from build123d import *

# Parameters (mm, degrees)
F0_W      = 57.15
F0_H      = 31.75
F1_DEPTH  = 38.1
F2_DEPTH  = 12.7
F4_DEPTH  = 12.7
F6_DEPTH  = 12.7
F8_DEPTH  = 38.101
F9_DEPTH  = 6.35
F10_DEPTH = 6.35
F11_DEPTH = 6.35
F12_DEPTH = 6.35


with BuildPart() as f1:
    # F0 (on Front) → F1 (new body)
    with BuildSketch(Plane.XZ):
        with Locations((28.575, 15.875)):
            Rectangle(F0_W, F0_H)
    extrude(amount=F1_DEPTH)

    # F2 (add): a face of the model
    f2_faces = [f1.faces().sort_by_distance(p)[0] for p in [
        (28.575, -38.1, 15.875),
    ]]
    extrude(f2_faces, amount=F2_DEPTH)

    # F3 (on face) → F4 (cut)
    with BuildSketch(Plane.XZ.offset(50.8)):
        Polygon((57.15, 31.75), (23.6781723797, 31.75), (35.8164422214, 0), (57.15, 0), align=None)
    extrude(amount=-F4_DEPTH, mode=Mode.SUBTRACT)

    # F5 (on face) → F6 (cut)
    with BuildSketch(Plane(origin=(0, 0, 0), x_dir=(-1, 0, 0), z_dir=(0, 1, 0))):
        Polygon((-33.819206059, 0), (-23.4500579536, 31.75), (-57.15, 31.75), (-57.15, 0), align=None)
    extrude(amount=-F6_DEPTH, mode=Mode.SUBTRACT)

    # F7 (on face) → F8 (cut, through all)
    with BuildSketch(Plane.XZ.offset(38.1)):
        Polygon((57.15, 31.75), (43.5097105801, 31.75), (57.15, 0), align=None)
    extrude(amount=-F8_DEPTH, mode=Mode.SUBTRACT)

    # F9 (cut): a face of the model
    f9_faces = [f1.faces().sort_by_distance(p)[0] for p in [
        (40.1169646518, -38.1, 15.6819192663),
    ]]
    extrude(f9_faces, amount=-F9_DEPTH, mode=Mode.SUBTRACT)

    # F10 (cut): a face of the model
    f10_faces = [f1.faces().sort_by_distance(p)[0] for p in [
        (39.6330799675, -12.7, 15.4760691102),
    ]]
    extrude(f10_faces, amount=-F10_DEPTH, mode=Mode.SUBTRACT)

    # F11 (cut): a face of the model
    f11_faces = [f1.faces().sort_by_distance(p)[0] for p in [
        (14.4737687914, 0, 14.9168931282),
    ]]
    extrude(f11_faces, amount=-F11_DEPTH, mode=Mode.SUBTRACT)

    # F12 (cut): a face of the model
    f12_faces = [f1.faces().sort_by_distance(p)[0] for p in [
        (15.0800275041, -50.8, 14.7953782839),
    ]]
    extrude(f12_faces, amount=-F12_DEPTH, mode=Mode.SUBTRACT)


solid = f1.part
Input: part model. Units: mm. Frame: model coordinates. A direction names the side the tool comes from. Coordinates: 2 decimals unless noted, no trailing zeros. Loops run counter-clockwise (first coordinate to the right, second up) from the corner with the lowest first, then second, coordinate; pieces in that order, holes last.
(1) Section D-D on y = -33. Return the cut outline in (x, z), then the cut area to 3 significant figures.
(2) Section A-A on z = 12.5. Return the cut outline in (x, y), then the cut area to 3 significant figures.
(3) Section C-C on z = 24.5. Return the cut outline in (x, y), then the cut area to 3 significant figures.
(4) First-contact query: pin 1 Ø5 at (x, y) = (48.5, -35.5) entering from -Z; pin 2 Ø9.5 at (x, z) = (41.5, 17.5) entering from +Y; pin 3 Ø2 at (y, z) = (-26, 26) entering from -X; pin 4 Ø9.5 at (x, z) = (35.5, 14.5) entering from -Y. Flat tips, straight axial feed; report the tip coordinate or a pass-through.
(5) Pull-direction query (Y, two-part tool) for faces 1 (the face through (41, -19.05, 16)), 2 (the face through (14, -44.45, 16)), 3 (the face through (17, -25, 31.75)); classes: released by +Y, released by -Y, zero draft, split by the parting line, or undercut.
(6) Section B-B on y = -17. Return the cut outline in (x, z).
(7) Material intervals for probe 1 along Y at (x, z) = (36, 3); probe 2 along X at (y, z) = (-35.5, 21.5), sorted ascending.
(8) Set-up query: faces 4 (the face through (22, -25, 0)), 5 (the face through (28.71, -12.61, 15.65)), 6 (the face through (29.66, -38.19, 16.1)). Return all of +Z, -Z, +X, -X, +Y, -Y with unobstructed straight access to the full face (end or side cutting, diameter ignored); none if empty.
Data:
1. outline: (0, 0) - (35.82, 0) - (23.68, 31.75) - (0, 31.75) - close
1. area: 944 mm2
2. outline: (0, -44.45) - (31.04, -44.45) - (31.04, -31.75) - (51.78, -31.75) - (51.78, -19.05) - (29.74, -19.05) - (29.74, -6.35) - (0, -6.35) - close
2. area: 1,430 mm2
3. outline: (0, -44.45) - (26.45, -44.45) - (26.45, -31.75) - (46.62, -31.75) - (46.62, -19.05) - (25.82, -19.05) - (25.82, -6.35) - (0, -6.35) - close
3. area: 1,260 mm2
4. pin 1: passes through
4. pin 2: stops at y = -19.05
4. pin 3: stops at x = 0
4. pin 4: stops at y = -31.75
5. face 1: released by +Y
5. face 2: released by -Y
5. face 3: zero draft
6. outline: (0, 0) - (33.82, 0) - (23.45, 31.75) - (0, 31.75) - close
7. probe 1: y = -31.75 to -19.05
7. probe 2: x = 0 to 27.6
8. face 4: -Z, +X, -X, +Y, -Y
8. face 5: +Z, +X, +Y
8. face 6: +Z, +X, -Y
